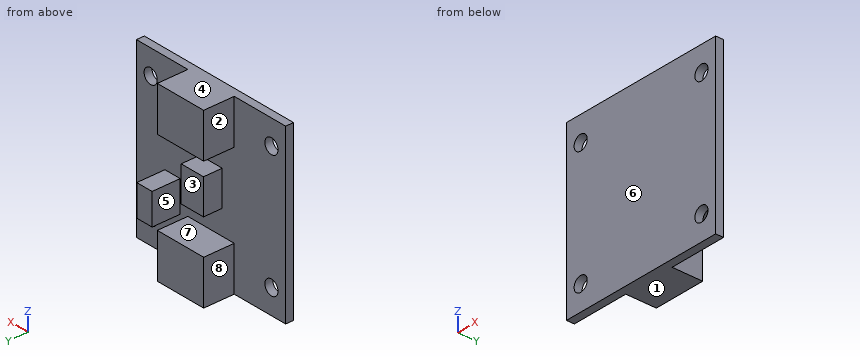
Autodesk Inventor part; units mm, degrees
ref_plane "YZ Plane" through (0, 0, 0) normal (1, 0, 0) x (0, 1, 0)
ref_plane "XZ Plane" through (0, 0, 0) normal (0, 1, 0) x (-1, 0, 0)
ref_plane "XY Plane" through (0, 0, 0) normal (0, 0, 1) x (1, 0, 0)
sketch "Skizze1" plane through (0, 0, 0) normal (0, 1, 0) x (-1, 0, 0)
  line L0 (17.05, 17.5) -> (-17.05, 17.5)
  line L1 (-17.05, 17.5) -> (-17.05, -17.5)
  line L2 (-17.05, -17.5) -> (17.05, -17.5)
  line L3 (17.05, -17.5) -> (17.05, 17.5)
  point P0 (0, 0)
  dimension "d0" = 35
  dimension "d1" = 34.1
  dimension "d2" = 17.5
  dimension "d3" = 17.05
extrude "Extrusion1" add sketch "Skizze1" along normal blind 1.6
sketch "Skizze3" plane through (0, 1.6, 0) normal (0, 1, 0) x (1, 0, 0)
  line L0 (-17.05, 17.5) -> (-17.05, -17.5)
  line L1 (17.05, -17.5) -> (17.05, 17.5)
  line L2 (-21.1922, 0) -> (21.294, 0)
  point P0 (0, 0)
  point P1 (-13.8, -12.5)
  point P2 (13.8, 12.5)
  point P3 (13.8, -12.5)
  point P4 (-13.8, 12.5)
  dimension "d13" = 3.25
  dimension "d15" = 3.25
  dimension "d16" = 25
  dimension "d18" = 25
hole "Bohrung2" at (-13.8, 1.6, 12.5) at (13.8, 1.6, -12.5) at (13.8, 1.6, 12.5) at (-13.8, 1.6, -12.5) direction (0, -1, 0) diameter 3 end through all
sketch "Skizze4" plane through (0, 1.6, 0) normal (0, 1, 0) x (1, 0, 0)
  line L0 (17.05, 17.5) -> (-17.05, 17.5)
  line L1 (-5.3, 17.5) -> (5.3, 17.5)
  line L2 (5.3, 17.5) -> (5.3, 8.5)
  line L3 (5.3, 8.5) -> (-5.3, 8.5)
  line L4 (-5.3, 8.5) -> (-5.3, 17.5)
  line L5 (0, -9.1387) -> (0, 30.8608)
  line L6 (-26.2563, 0) -> (26.186, 0)
  line L7 (-17.05, -17.5) -> (17.05, -17.5)
  line L8 (-5.3, -17.5) -> (5.3, -17.5)
  line L9 (5.3, -17.5) -> (5.3, -8.5)
  line L10 (5.3, -8.5) -> (-5.3, -8.5)
  line L11 (-5.3, -8.5) -> (-5.3, -17.5)
  point P0 (0, 0)
  dimension "d26" = 9
  dimension "d27" = 10.6
extrude "Extrusion2" add sketch "Skizze4" along normal blind 6.2
sketch "Skizze5" plane through (0, 1.6, 0) normal (0, 1, 0) x (1, 0, 0)
  line L0 (10.55, 2.6) -> (7.05, 2.6)
  line L1 (7.05, 2.6) -> (7.05, 8.9)
  line L2 (7.05, 8.9) -> (10.55, 8.9)
  line L3 (10.55, 8.9) -> (10.55, 2.6)
  line L4 (17.05, -17.5) -> (17.05, 17.5)
  line L5 (17.05, 17.5) -> (5.3, 17.5)
  point P0 (0, 0)
  dimension "d32" = 6.3
  dimension "d33" = 3.5
  dimension "d34" = 6.5
  dimension "d35" = 8.6
extrude "Extrusion3" add sketch "Skizze5" along normal blind 5.7
sketch "Skizze6" plane through (0, 1.6, 0) normal (0, 1, 0) x (1, 0, 0)
  line L0 (-2.55, -3.55) -> (2.55, -3.55)
  line L1 (2.55, -3.55) -> (2.55, 3.55)
  line L2 (2.55, 3.55) -> (-2.55, 3.55)
  line L3 (-2.55, 3.55) -> (-2.55, -3.55)
  line L4 (-17.05, 17.5) -> (-17.05, -17.5)
  line L5 (5.3, 17.5) -> (-5.3, 17.5)
  point P0 (0, 0)
  dimension "d38" = 7.1
  dimension "d39" = 5.1
  dimension "d40" = 14.5
  dimension "d41" = 13.95
extrude "Extrusion4" add sketch "Skizze6" along normal blind 3.8
properties part number "Prozessorboard"
Part model, mm, in its own coordinate system. Face numbers are marked on the shaded views. A direction names the side the tool comes from. Round coordinates to 2 decimals unless told otherwise and drop trailing zeros. Write each loop counter-clockwise with the first axis right and the second up, starting at its lowest first coordinate (ties: lowest second). Pieces come first, ordered by that corner, then holes. Notation, with made-up numbers: (-5, -8) - (4, -8) arc R26 cw to (4, 16) - close; hole circle Ø3 at (57, 2.5). An arc over 180 degrees is marked (long way). Use CSV: the item, a comma, the result in double quotes.
Item 1: Slice it at D-D, the plane x = -13.8. Write the cut outline in (y, z), then the cut area to 3 significant figures.
Results list:
outline,"(0, -17.5) - (1.6, -17.5) - (1.6, -14) - (0, -14) - close; (0, -11) - (1.6, -11) - (1.6, 11) - (0, 11) - close; (0, 14) - (1.6, 14) - (1.6, 17.5) - (0, 17.5) - close"
area,"46.4 mm²"
Item 2: Flat gauge pins, fed straight in: P1, Ø2.5, axis at x = 13.8, z = -12.5, coming from the +Y side; P2, Ø1.9, axis at y = 6, z = -11, coming from the -X side; P3, Ø4, axis at x = -12, z = 1, coming from the +Y side; P4, Ø3, axis at y = 3.5, z = 13.5, coming from the +X side. Where does each tip first touch, or does it go through?
Results list:
P1,"passes through"
P2,"stops at x = -5.3"
P3,"stops at y = 1.6"
P4,"stops at x = 5.3"
Item 3: Pull direction Z, two halves, no side cores. Call the marked faces 1, 2, 3 and 4: pulls with the +Z half, pulls with the -Z half, needs draft (parallel to the pull), parting line crosses it, or undercut.
Results list:
face 1,"pulls with the -Z half"
face 2,"needs draft"
face 3,"undercut"
face 4,"pulls with the +Z half"
Item 4: Slice it at C-C, the plane y = 4.5. Write the cut outline in (x, z).
Results list:
outline,"(-5.3, -17.5) - (5.3, -17.5) - (5.3, -8.5) - (-5.3, -8.5) - close; (-5.3, 8.5) - (5.3, 8.5) - (5.3, 17.5) - (-5.3, 17.5) - close; (-2.55, -3.55) - (2.55, -3.55) - (2.55, 3.55) - (-2.55, 3.55) - close; (7.05, -8.9) - (10.55, -8.9) - (10.55, -2.6) - (7.05, -2.6) - close"
Item 5: Tool access for the marked faces 5, 6, 7 and 8: list every direction of +Z, -Z, +X, -X, +Y, -Y with a clear straight run to the whole face (end or side of a thin tool).
Results list:
face 5,"+Z, -Z, +Y"
face 6,"+Z, -Z, +X, -X, -Y"
face 7,"-X, +Y"
face 8,"+Z, -Z, -X, +Y"
Item 6: Slice it at B-B, the plane z = -12.5. Write the cut outline in (x, y), then the cut area to 3 significant figures.
Results list:
outline,"(-17.05, 0) - (-15.3, 0) - (-15.3, 1.6) - (-17.05, 1.6) - close; (-12.3, 0) - (12.3, 0) - (12.3, 1.6) - (5.3, 1.6) - (5.3, 7.8) - (-5.3, 7.8) - (-5.3, 1.6) - (-12.3, 1.6) - close; (15.3, 0) - (17.05, 0) - (17.05, 1.6) - (15.3, 1.6) - close"
area,"111 mm²"
Item 7: Wall check: L1, parallel to Z at x = 13.8, y = 0.7; L2, parallel to X at y = 0.45, z = -12.5; L3, parallel to Z at x = -2, y = 1.75. Give the ranges that are in metal, low to high.
Results list:
L1,"z = -17.5 to -14, -11 to 11, 14 to 17.5"
L2,"x = -17.05 to -15.3, -12.3 to 12.3, 15.3 to 17.05"
L3,"z = -17.5 to -8.5, -3.55 to 3.55, 8.5 to 17.5"
Item 8: Slice it at A-A, the plane y = 1. Write the cut outline in (x, z), then the cut area to 3 significant figures.
Results list:
outline,"(-17.05, -17.5) - (17.05, -17.5) - (17.05, 17.5) - (-17.05, 17.5) - close; hole circle Ø3 at (-13.8, -12.5); hole circle Ø3 at (-13.8, 12.5); hole circle Ø3 at (13.8, -12.5); hole circle Ø3 at (13.8, 12.5)"
area,"1,170 mm²"
